Input: part model. Units: mm. Frame: model coordinates. A direction names the side the tool comes from. Coordinates: 2 decimals unless noted, no trailing zeros. Write each loop counter-clockwise with the first axis right and the second up, starting at its lowest first coordinate (ties: lowest second). Pieces come first, ordered by that corner, then holes. Notation, with made-up numbers: M -2,-2 L 12,-2 A16 ccw 12,27 Z; hole C 24,37.5 d5. An arc over 180 degrees is marked long. Use one line per item in the form item = value.
from build123d import *

# Parameters (mm, degrees)
F3_START = -8.89
F2_R     = 4.826
F3_DEPTH = 92.71
F4_R     = 3.175
F5_DEPTH = 41.148


with BuildPart() as f1:
    # F0 (on Front) → F1 (revolve)
    with BuildSketch(Plane.XZ):
        with BuildLine():
            Line((-6.35, 0), (0, 0))
            Line((0, 0), (0, 12.7))
            Line((0, 12.7), (-6.35, 12.7))
            Line((-6.35, 12.7), (-6.3650681608, 12.7))
            ThreePointArc((-6.3650681608, 12.7), (-7.3377104297, 10.9657874542), (-9.2615922964, 10.4635875931))
            Line((-9.2615922964, 10.4635875931), (-24.384, 12.7))
            Line((-24.384, 12.7), (-33.274, 12.7))
            Line((-33.274, 12.7), (-60.9909756098, 12.7))
            Line((-60.9909756098, 12.7), (-69.8809756098, 12.7))
            Line((-69.8809756098, 12.7), (-99.4210244843, 12.7))
            ThreePointArc((-99.4210244843, 12.7), (-101.0513051228, 6.4427853895), (-101.6, 0))
            Line((-101.6, 0), (-6.35, 0))
        make_face()
    revolve(axis=Axis((-50.8, 0, 0), (-1, 0, 0)))

    # F2 (on Right) → F3 (cut)
    with BuildSketch(Plane.YZ.offset(F3_START)):
        with Locations((-16.002, 0)):
            Circle(F2_R)
        with Locations((-8.001, 13.8581385114)):
            Circle(F2_R)
        with Locations((8.001, 13.8581385114)):
            Circle(F2_R)
        with Locations((16.002, 0)):
            Circle(F2_R)
        with Locations((8.001, -13.8581385114)):
            Circle(F2_R)
        with Locations((-8.001, -13.8581385114)):
            Circle(F2_R)
    extrude(amount=-F3_DEPTH, mode=Mode.SUBTRACT)

    # F4 (on Right) → F5 (cut)
    with BuildSketch(Plane.YZ):
        Circle(F4_R)
    extrude(amount=-F5_DEPTH, mode=Mode.SUBTRACT)


solid = f1.part
(1) Section query B-B on z = 0. Return the cut outline in (x, y) (3 decimals).
Computed:
outline = M -99.924,-11.176 L -14.079,-11.176 L -9.262,-10.464 A2.54 cw -6.365,-12.7 L 0,-12.7 L 0,-3.175 L -41.148,-3.175 L -41.148,3.175 L 0,3.175 L 0,12.7 L -6.365,12.7 A2.54 cw -9.262,10.464 L -14.079,11.176 L -99.924,11.176 A38.1 ccw Z
(2) Section query C-C on x = -20. Return the cut outline in (y, z) (3 decimals), plus the area to 3 significant figures.
Computed:
outline = M -11.812,-2.394 A12.052 ccw -7.979,-9.032 A4.826 cw -3.833,-11.426 A12.052 ccw 3.833,-11.426 A4.826 cw 7.979,-9.032 A12.052 ccw 11.812,-2.394 A4.826 cw 11.812,2.394 A12.052 ccw 7.979,9.032 A4.826 cw 3.833,11.426 A12.052 ccw -3.833,11.426 A4.826 cw -7.979,9.032 A12.052 ccw -11.812,2.394 A4.826 cw Z; hole C 0,0 d6.35
area = 408 mm^2
(3) Section query D-D on y = 0. Return the cut outline in (x, z) (3 decimals).
Computed:
outline = M -99.421,-12.7 L -24.384,-12.7 L -9.262,-10.464 A2.54 cw -6.365,-12.7 L 0,-12.7 L 0,-3.175 L -41.148,-3.175 L -41.148,3.175 L 0,3.175 L 0,12.7 L -6.365,12.7 A2.54 cw -9.262,10.464 L -24.384,12.7 L -99.421,12.7 A38.1 ccw Z
(4) Pull-direction query (Z, two-part tool) for faces 1 (the cylindrical face through (-62.428, 10.974, 6.392)), 2 (the cylindrical face through (-20.29, -0.69, -3.1)), 3 (the cylindrical face through (-3.23, -12.4, -2.75)), 4 (the cylindrical face through (-62.43, 11.02, -6.31)); classes: pulls with the +Z half, pulls with the -Z half, needs draft (parallel to the pull), parting line crosses it, or undercut.
Computed:
face_1 = pulls with the +Z half
face_2 = undercut
face_3 = parting line crosses it
face_4 = pulls with the -Z half
(5) Line query: probe 1 along Z at (x, y) = (-30, 0) (3 decimals); probe 2 along Z at (x, y) = (-12, 0) (3 decimals); probe 3 along Z at (x, y) = (-44.5, 0). Output: solid intervals per line, ascending.
Computed:
probe_1 = -12.7 to -3.175, 3.175 to 12.7
probe_2 = -10.869 to -3.175, 3.175 to 10.869
probe_3 = -12.7 to 12.7
(6) Set-up query: faces 5 (the cylindrical face through (-56.399, 11.176, 0.047)), 6 (the flat face through (-41.148, 0, 0)), 7 (the cylindrical face through (-56.391, -11.176, -0.047)). Return all of +Z, -Z, +X, -X, +Y, -Y with unobstructed straight access to the full face (end or side cutting, diameter ignored); none if empty.
Computed:
face_5 = -X, +Y
face_6 = +X
face_7 = -X, -Y
(7) Section query A-A on x = -87.5. Return the cut outline in (y, z).
Computed:
outline = M -12.31,-3.11 A12.7 ccw -8.85,-9.11 A4.83 cw -3.46,-12.22 A12.7 ccw 3.46,-12.22 A4.83 cw 8.85,-9.11 A12.7 ccw 12.31,-3.11 A4.83 cw 12.31,3.11 A12.7 ccw 8.85,9.11 A4.83 cw 3.46,12.22 A12.7 ccw -3.46,12.22 A4.83 cw -8.85,9.11 A12.7 ccw -12.31,3.11 A4.83 cw Z
(8) First-contact query: pin 1 Ø4 at (x, z) = (-21, 3.5) entering from +Y; pin 2 Ø12 at (y, z) = (-5.5, 7) entering from -X; pin 3 Ø12 at (x, y) = (-18.5, 8.5) entering from -Z. Flat tips, straight axial feed; report the tip coordinate or a pass-through.
Computed:
pin_1 = 12.14
pin_2 = -101.49
pin_3 = -11.82
